```python
from build123d import *

# Parameters (mm, degrees)
BOSS_EXTRUDE1_DEPTH = 36
FILLET1_R           = 2.5
SKETCH2_R           = 10
BOSS_EXTRUDE2_DEPTH = 4
SKETCH3_R           = 5
BOSS_EXTRUDE3_DEPTH = 10
FILLET2_R           = 1


with BuildPart() as part:
    # Sketch1 → Boss-Extrude1 (new body)
    with BuildSketch(Plane(origin=(0, 0, 0), x_dir=(1, 0, 0), z_dir=(0, 1, 0))):
        with BuildLine():
            Line((66.5, -98), (-66.5, -98))
            ThreePointArc((-66.5, -98), (-68.267766953, -97.267766953), (-69, -95.5))
            Line((-69, -95.5), (-69, 95.5))
            ThreePointArc((-69, 95.5), (-68.267766953, 97.267766953), (-66.5, 98))
            Line((-66.5, 98), (66.5, 98))
            ThreePointArc((66.5, 98), (68.267766953, 97.267766953), (69, 95.5))
            Line((69, 95.5), (69, -95.5))
            ThreePointArc((69, -95.5), (68.267766953, -97.267766953), (66.5, -98))
        make_face()
    extrude(amount=BOSS_EXTRUDE1_DEPTH)

    # Fillet1
    fillet1_edges = [part.edges().sort_by_distance(p)[0] for p in [
        (69, 0, 0),
        (68.267766953, 0, 97.267766953),
        (0, 0, 98),
        (-68.267766953, 0, 97.267766953),
        (68.267766953, 36, 97.267766953),
        (69, 36, 0),
        (68.267766953, 36, -97.267766953),
        (0, 36, -98),
        (-68.267766953, 36, -97.267766953),
        (-69, 36, 0),
        (-68.267766953, 36, 97.267766953),
        (-69, 0, 0),
        (0, 36, 98),
        (-68.267766953, 0, -97.267766953),
        (0, 0, -98),
        (68.267766953, 0, -97.267766953),
    ]]
    fillet(fillet1_edges, radius=FILLET1_R)

    # Sketch2 → Boss-Extrude2 (add)
    with BuildSketch(Plane(origin=(0, 0, -98), x_dir=(-1, 0, 0), z_dir=(0, 0, -1))):
        with Locations(Location((-37.5, 18, 0), (0, 0, 180))):
            Circle(SKETCH2_R)
        with Locations(Location((37.5, 18, 0), (0, 0, 180))):
            Circle(SKETCH2_R)
    extrude(amount=BOSS_EXTRUDE2_DEPTH)

    # Sketch3 → Boss-Extrude3 (add)
    with BuildSketch(Plane(origin=(0, 0, -102), x_dir=(-1, 0, 0), z_dir=(0, 0, -1))):
        with Locations((-37.5, 18)):
            Circle(SKETCH3_R)
        with Locations((37.5, 18)):
            Circle(SKETCH3_R)
    extrude(amount=BOSS_EXTRUDE3_DEPTH)

    # Fillet2
    fillet2_edges = [part.edges().sort_by_distance(p)[0] for p in [
        (27.5, 18, -102),
        (-47.5, 18, -102),
        (42.5, 18, -112),
        (-32.5, 18, -112),
    ]]
    fillet(fillet2_edges, radius=FILLET2_R)


solid = part.part
```
Geometry check sheet. Reference: the model listing, model coordinates, mm. A direction names the side the tool comes from. Coordinates: 2 decimals unless noted, no trailing zeros. Loops run counter-clockwise (first coordinate to the right, second up) from the corner with the lowest first, then second, coordinate; pieces in that order, holes last.
Item 1: Thickness scan on line 1 (Z direction, x = 5.5, y = 5); line 2 (Z direction, x = -30.5, y = 17); line 3 (X direction, y = 34, z = -70). Record the ranges inside material, lowest first.
Item 2: Release check for a two-part mould opening along X. For faces 1 (the face through (1, 0, -1)), 2 (the face through (-69, 18, 1)), 3 (the face through (36.198, 8.085, -99.479)) record: released by +X, released by -X, zero draft, split by the parting line, or undercut.
Item 3: Sectioned sample at C-C, the plane y = 30.5. Record the boundary of the cut face in (x, z).
Item 4: Sectioned sample at D-D, the plane x = -50.5. Record the boundary of the cut face in (y, z).
Item 5: Access from +Z, -Z, +X, -X, +Y, -Y to the whole of each face (thin tool, end or side, straight path). Record for faces 4 (the face through (-34, 22, -102)), 5 (the face through (1, 36, -1)).
Item 6: Go/stop test with a flat-tipped pin: pin 1 Ø8 at (x, y) = (0, 7.5) entering from -Z. Record where the tip stops, or that it passes through.
Item 7: Sectioned sample at B-B, the plane x = 37.5. Record the boundary of the cut face in (y, z).
Check result:
1. line 1: z = -98 to 98
1. line 2: z = -102 to 98
1. line 3: x = -68.95 to 68.95
2. face 1: zero draft
2. face 2: released by -X
2. face 3: undercut
3. outline: (-69, -95.5) arc R2.5 ccw to (-66.5, -98) - (66.5, -98) arc R2.5 ccw to (69, -95.5) - (69, 95.5) arc R2.5 ccw to (66.5, 98) - (-66.5, 98) arc R2.5 ccw to (-69, 95.5) - close
4. outline: (0, -95.5) arc R2.5 ccw to (2.5, -98) - (33.5, -98) arc R2.5 ccw to (36, -95.5) - (36, 95.5) arc R2.5 ccw to (33.5, 98) - (2.5, 98) arc R2.5 ccw to (0, 95.5) - close
5. face 4: -Z
5. face 5: +Z, -Z, +X, -X, +Y
6. pin 1: stops at z = -98
7. outline: (0, -95.5) arc R2.5 ccw to (2.5, -98) - (8, -98) - (8, -101) arc R1 ccw to (9, -102) - (13, -102) - (13, -111) arc R1 ccw to (14, -112) - (22, -112) arc R1 ccw to (23, -111) - (23, -102) - (27, -102) arc R1 ccw to (28, -101) - (28, -98) - (33.5, -98) arc R2.5 ccw to (36, -95.5) - (36, 95.5) arc R2.5 ccw to (33.5, 98) - (2.5, 98) arc R2.5 ccw to (0, 95.5) - close
